from build123d import *

# Parameters (mm, degrees)
EXTRU_MINCE1_DEPTH      = 84
ESQUISSE2_R             = 1.5
ENL_V_MAT_EXTRU_1_DEPTH = 8
ESQUISSE3_R             = 1.5
ESQUISSE3_W             = 25.5
ESQUISSE3_H             = 40
ENL_V_MAT_EXTRU_2_DEPTH = 5
ESQUISSE4_W             = 5.5
ESQUISSE4_H             = 84
ENL_V_MAT_EXTRU_3_DEPTH = 6
CHANFREIN1_SIZE         = 17
CHANFREIN1_SIZE2        = 23
CONG_1_R                = 5


with BuildPart() as part:
    # Esquisse1 → Extru.-Mince1 (new body)
    with BuildSketch(Plane.XY):
        Polygon((0, 15.5), (0, 0), (27.5, 0), (27.5, 1.5), (1.5, 1.5), (1.5, 15.5), align=None)
    extrude(amount=EXTRU_MINCE1_DEPTH)

    # Esquisse2 → Enlèv. mat.-Extru.1 (cut)
    with BuildSketch(Plane.ZY):
        with Locations(Location((7, 7.5, 0), (0, 0, 270))):
            Circle(ESQUISSE2_R)
        with Locations(Location((24, 7.5, 0), (0, 0, 270))):
            Circle(ESQUISSE2_R)
        with Locations(Location((60, 7.5, 0), (0, 0, 270))):
            Circle(ESQUISSE2_R)
        with Locations(Location((77, 7.5, 0), (0, 0, 90))):
            Circle(ESQUISSE2_R)
    extrude(amount=-ENL_V_MAT_EXTRU_1_DEPTH, mode=Mode.SUBTRACT)

    # Esquisse3 → Enlèv. mat.-Extru.2 (cut)
    with BuildSketch(Plane.XZ):
        with Locations(Location((7, 56, 0), (0, 0, 270))):
            Circle(ESQUISSE3_R)
        with Locations(Location((17, 56, 0), (0, 0, 270))):
            Circle(ESQUISSE3_R)
        with Locations(Location((17, 8, 0), (0, 0, 90))):
            Circle(ESQUISSE3_R)
        with Locations(Location((7, 8, 0), (0, 0, 90))):
            Circle(ESQUISSE3_R)
        with Locations((14.75, 32)):
            Rectangle(ESQUISSE3_W, ESQUISSE3_H)
    extrude(amount=-ENL_V_MAT_EXTRU_2_DEPTH, mode=Mode.SUBTRACT)

    # Esquisse4 → Enlèv. mat.-Extru.3 (cut)
    with BuildSketch(Plane.XZ):
        with Locations((24.75, 42)):
            Rectangle(ESQUISSE4_W, ESQUISSE4_H)
    extrude(amount=-ENL_V_MAT_EXTRU_3_DEPTH, mode=Mode.SUBTRACT)

    # Chanfrein1
    chanfrein1_edges = [part.edges().sort_by_distance(p)[0] for p in [
        (22, 0.75, 84),
    ]]
    chanfrein1_side = [part.faces().sort_by_distance(p)[0] for p in [
        (0.75, 15.230881067, 84),
    ]]
    chamfer(chanfrein1_edges, length=CHANFREIN1_SIZE, length2=CHANFREIN1_SIZE2, reference=chanfrein1_side[0])

    # Congé1
    cong_1_edges = [part.edges().sort_by_distance(p)[0] for p in [
        (22, 0.75, 61),
        (5, 0.75, 84),
        (0.75, 15.5, 84),
        (0.75, 15.5, 0),
        (22, 0.75, 0),
    ]]
    fillet(cong_1_edges, radius=CONG_1_R)


solid = part.part
Could you check a few things on this model? Use its own coordinates, in mm. A direction names the side the tool comes from. Give positions to 0.01 mm unless a question says otherwise; leave off trailing zeros. Write each loop counter-clockwise with the first axis right and the second up, starting at its lowest first coordinate (ties: lowest second). Pieces come first, ordered by that corner, then holes. Notation, with made-up numbers: (71.25, -14.5) - (87.25, -14.5) arc R19 cw to (87.25, 15.5) - close; hole circle Ø5 at (85, 13). An arc over 180 degrees is marked (long way). Use CSV: the item, a comma, the result in double quotes. Start each with the question number.
Item 1: I want a section at A-A, the plane z = 24. Please give me the cut outline in (x, y).
Item 2: I want a section at C-C, the plane x = 12.5. Please give me the cut outline in (y, z).
Item 3: If I drill on line 1 along Z through (x, y) = (0.5, 7.5); line 2 along X through (y, z) = (0.75, 8); line 3 along Z through (x, y) = (7.5, 1.25), over which ranges is the centre line in solid material (lowest first)?
Item 4: For faces 1 (the face through (12, 1, 52)), 2 (the face through (1.5, 8, 41)), 3 (the face through (22, 1, 56)), which set-ups out of +Z, -Z, +X, -X, +Y, -Y let a thin tool reach every point of the face, with its end or its side?
Item 5: If we mould it in two halves opening along Z, with no side actions, what happens to faces 4 (the face through (0.74, 7.695, 25.487)), 5 (the face through (1, 5, 84)), 6 (the face through (0.74, 7.305, 75.513)), 7 (the face through (20, 1, 1))? For each: pulls with the +Z half, pulls with the -Z half, needs draft (parallel to the pull), parting line crosses it, or undercut.
Item 6: I want a section at D-D, the plane z = 56. Please give me the cut outline in (x, y).
Item 7: I'm going to push flat-ended pins straight in: pin 1 (2.5 mm diameter, centred on y = 7.5, z = 7, fed in from +X); pin 2 (5 mm diameter, centred on y = 8, z = 32.5, fed in from +X); pin 3 (5 mm diameter, centred on x = 17, z = 56, fed in from +Y); pin 4 (1.2 mm diameter, centred on y = 1, z = 39.5, fed in from +X). Where does each tip first touch, or does it pass through?
Item 8: I want a section at B-B, the plane y = 7.5. Please give me the cut outline in (x, z).
Findings:
1,outline,"(0, 0) - (2, 0) - (2, 1.5) - (1.5, 1.5) - (1.5, 6) - (0, 6) - close; (0, 9) - (1.5, 9) - (1.5, 15.5) - (0, 15.5) - close"
2,outline,"(0, 0) - (1.5, 0) - (1.5, 12) - (0, 12) - close; (0, 52) - (1.5, 52) - (1.5, 73.85) - (0, 73.85) - close"
3,line 1,"z = 0 to 5.5, 8.5 to 22.5, 25.5 to 58.5, 61.5 to 75.5, 78.5 to 84"
3,line 2,"x = 0 to 5.5, 8.5 to 15.5, 18.5 to 22"
3,line 3,"z = 0 to 6.59, 9.41 to 12, 52 to 54.59, 57.41 to 80.62"
4,face 1,"+X, +Y, -Y"
4,face 2,"+Z, -Z, +X, +Y"
4,face 3,"+Z, -Z, +X, +Y, -Y"
5,face 4,"undercut"
5,face 5,"pulls with the +Z half"
5,face 6,"undercut"
5,face 7,"pulls with the -Z half"
6,outline,"(0, 0) - (5.5, 0) - (5.5, 1.5) - (1.5, 1.5) - (1.5, 15.5) - (0, 15.5) - close; (8.5, 0) - (15.5, 0) - (15.5, 1.5) - (8.5, 1.5) - close; (18.5, 0) - (22, 0) - (22, 1.5) - (18.5, 1.5) - close"
7,pin 1,"passes through"
7,pin 2,"stops at x = 1.5"
7,pin 3,"stops at y = 1.5"
7,pin 4,"stops at x = 2"
8,outline,"(0, 0) - (1.5, 0) - (1.5, 5.5) - (0, 5.5) - close; (0, 8.5) - (1.5, 8.5) - (1.5, 22.5) - (0, 22.5) - close; (0, 25.5) - (1.5, 25.5) - (1.5, 58.5) - (0, 58.5) - close; (0, 61.5) - (1.5, 61.5) - (1.5, 75.5) - (0, 75.5) - close; (0, 78.5) - (1.5, 78.5) - (1.5, 84) - (0, 84) - close"
